Study the drawing (mm; zero at the part's minimum x, y, z) and answer. A direction names the side the tool comes from. Coordinates: 2 decimals unless noted, no trailing zeros. Write each loop counter-clockwise with the first axis right and the second up, starting at its lowest first coordinate (ties: lowest second). Pieces come first, ordered by that corner, then holes. Notation, with made-up numbers: (56, 77.5) - (80, 77.5) arc R28 ccw to (80, 103.5) - close; hole circle Ø1 at (75, 10). An arc over 180 degrees is marked (long way). One line per item, written item: value.
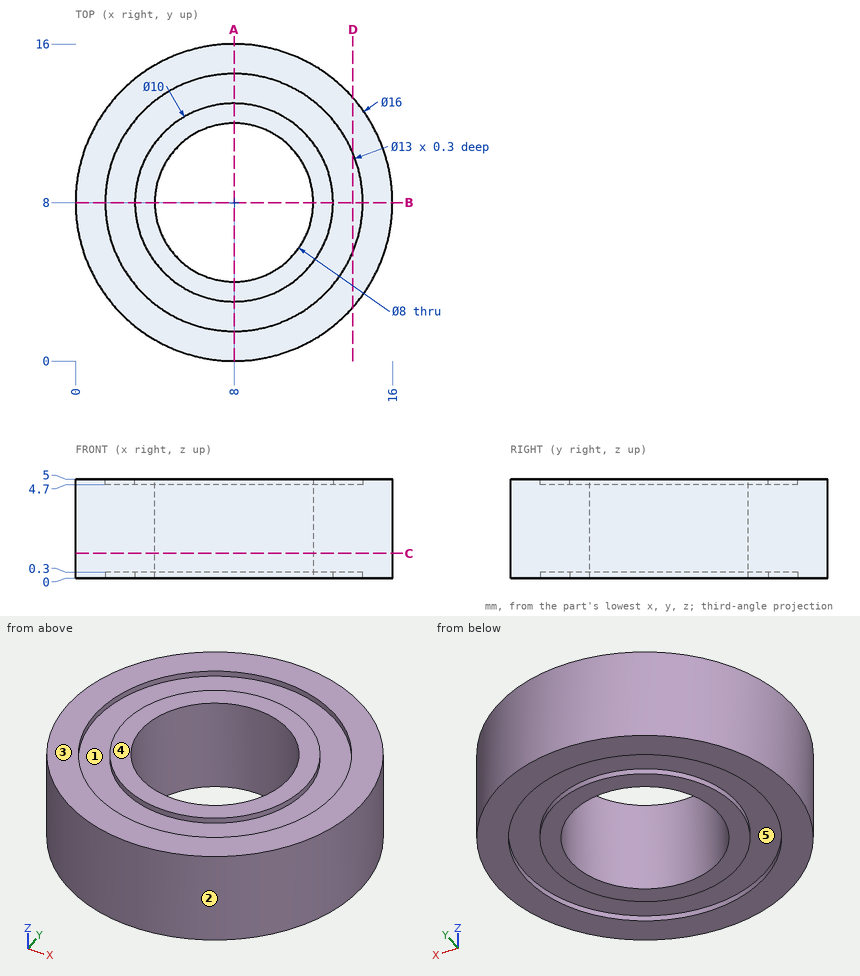
Item 1: Given pin 1 (8 mm diameter, centred on x = 11.5, y = 6, fed in from -Z); pin 2 (1.5 mm diameter, centred on x = 5, z = 3, fed in from -Y); pin 3 (3 mm diameter, centred on x = 10, z = 3.5, fed in from +Y); pin 4 (3 mm diameter, centred on x = 3.5, z = 0.5, fed in from +Y), each flat-ended and moving along its own axis, determine where each tip first touches the part or whether it passes through.
Evaluation:
pin 1: stops at z = 0
pin 2: stops at y = 0.32
pin 3: stops at y = 15.98
pin 4: stops at y = 15.42
Item 2: Section C-C, the plane z = 1.25 is taken. Determine the outline of the cut face in (x, y), then the cut area to 3 significant figures.
Evaluation:
outline: circle Ø16 at (8, 8); hole circle Ø8 at (8, 8)
area: 151 mm2
Item 3: Which of the six approach directions +Z, -Z, +X, -X, +Y, -Y give full straight-line access (tool end or side, diameter ignored) to the marked faces 4 and 5?
Evaluation:
face 4: +Z, +X, -X, +Y, -Y
face 5: -Z
Item 4: Consider probe 1 along Y at (x, z) = (8, 4.85); probe 2 along Y at (x, z) = (8, 3.65); probe 3 along X at (y, z) = (7.75, 2.4). Determine where each line is inside the solid, lowest interval first.
Evaluation:
probe 1: y = 0 to 1.5, 3 to 4, 12 to 13, 14.5 to 16
probe 2: y = 0 to 4, 12 to 16
probe 3: x = 0 to 4.01, 11.99 to 16
Item 5: Determine the mould class of the marked faces 1, 2 and 3 for opening direction X: +X half, -X half, draft (parallel to the pull), parting line (faces both ways), or undercut.
Evaluation:
face 1: undercut
face 2: parting line
face 3: draft
Item 6: Section D-D, the plane x = 14 is taken. Determine the outline of the cut face in (y, z).
Evaluation:
outline: (2.71, 0) - (5.5, 0) - (5.5, 0.3) - (10.5, 0.3) - (10.5, 0) - (13.29, 0) - (13.29, 5) - (10.5, 5) - (10.5, 4.7) - (5.5, 4.7) - (5.5, 5) - (2.71, 5) - close
Item 7: Section A-A, the plane x = 8 is taken. Determine the outline of the cut face in (y, z), then the cut area to 3 significant figures.
Evaluation:
outline: (0, 0) - (1.5, 0) - (1.5, 0.3) - (3, 0.3) - (3, 0) - (4, 0) - (4, 5) - (3, 5) - (3, 4.7) - (1.5, 4.7) - (1.5, 5) - (0, 5) - close; (12, 0) - (13, 0) - (13, 0.3) - (14.5, 0.3) - (14.5, 0) - (16, 0) - (16, 5) - (14.5, 5) - (14.5, 4.7) - (13, 4.7) - (13, 5) - (12, 5) - close
area: 38.2 mm2
